Can you work these out from the drawing? Everything is in mm from the part's minimum corner. A direction names the side the tool comes from. Coordinates: 2 decimals unless noted, no trailing zeros. Write each loop counter-clockwise with the first axis right and the second up, starting at its lowest first coordinate (ties: lowest second). Pieces come first, ordered by that corner, then holes.
(1) Imagine slicing it at C-C, the plane x = 3.5. List the corners of the cut face in (y, z) for me.
(2) Imagine slicing it at A-A, the plane y = 29.95. List the corners of the cut face in (x, z) for me.
(3) For pin 1 Ø3 at (x, z) = (8.5, 10) entering from -Y; pin 2 Ø1.4 at (x, y) = (6, 2.25) entering from -Z; pin 3 Ø1.3 at (x, y) = (8, 2) entering from -Z; pin 4 Ø2.5 at (x, z) = (4, 20.5) entering from +Y, each with a flat end and sliding along its axis, tell me the tip position at first contact or that it passes through.
(4) Which directions (+Z, -Z, +X, -X, +Y, -Y) give clear straight access to the entire face, cutting with the end or side of a thin tool? Please do the marked faces 1, 2 and 3.
(5) Imagine slicing it at B-B, the plane z = 20.5. List the corners of the cut face in (x, y) for me, plus the area to 3 significant figures.
(6) Please list where these lines run through material, in increasing order: probe 1 along Y at (x, z) = (6, 17.55); probe 2 along Y at (x, z) = (6, 19.75); probe 3 along Z at (x, y) = (9.5, 22).
(7) Imagine slicing it at D-D, the plane y = 14. List the corners of the cut face in (x, z) for me, plus the area to 3 significant figures.
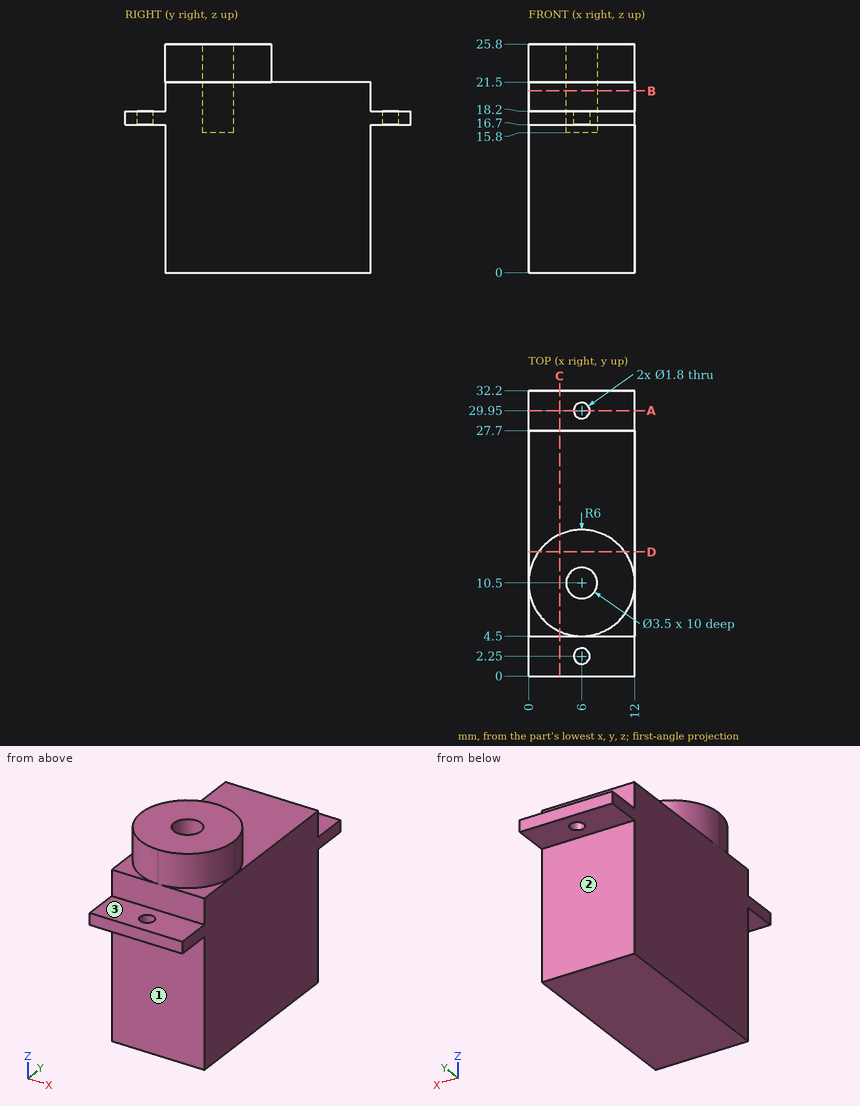
Recorded:
1. outline: (0, 16.7) - (4.5, 16.7) - (4.5, 0) - (27.7, 0) - (27.7, 16.7) - (32.2, 16.7) - (32.2, 18.2) - (27.7, 18.2) - (27.7, 21.5) - (15.95, 21.5) - (15.95, 25.8) - (5.05, 25.8) - (5.05, 21.5) - (4.5, 21.5) - (4.5, 18.2) - (0, 18.2) - close
2. outline: (0, 16.7) - (5.1, 16.7) - (5.1, 18.2) - (0, 18.2) - close; (6.9, 16.7) - (12, 16.7) - (12, 18.2) - (6.9, 18.2) - close
3. pin 1: stops at y = 4.5
3. pin 2: passes through
3. pin 3: stops at z = 16.7
3. pin 4: stops at y = 27.7
4. face 1: -Z, +X, -X, -Y
4. face 2: -Z, +X, -X, +Y
4. face 3: +Z, +X, -X, -Y
5. outline: (0, 4.5) - (12, 4.5) - (12, 27.7) - (0, 27.7) - close; hole circle Ø3.5 at (6, 10.5)
5. area: 269 mm2
6. probe 1: y = 0 to 1.35, 3.15 to 8.75, 12.25 to 29.05, 30.85 to 32.2
6. probe 2: y = 4.5 to 8.75, 12.25 to 27.7
6. probe 3: z = 0 to 21.5
7. outline: (0, 0) - (12, 0) - (12, 21.5) - (10.87, 21.5) - (10.87, 25.8) - (1.13, 25.8) - (1.13, 21.5) - (0, 21.5) - close
7. area: 300 mm2
